CAD build for the part. Positions are in the model's coordinates, mm. Face numbers are marked on the shaded views. Round coordinates to 2 decimals unless told otherwise and drop trailing zeros. Loops run counter-clockwise (first coordinate to the right, second up) from the corner with the lowest first, then second, coordinate; pieces in that order, holes last. Notation, with made-up numbers: M 69.25,27 L 87.25,27 A16 ccw 87.25,32 Z; hole C 49.5,-28 d8. An arc over 180 degrees is marked long. Use a Markdown table: item, result. Add a question column.
(1) Band-saw the part on B-B, the plane y = 19. Write the cut outline in (x, z) (3 decimals), and give its area (3 significant figures).
(2) Wall check: L1, parallel to Y at x = -1, z = -1.5 (3 decimals); L2, parallel to Y at x = 0, z = -3.5; L3, parallel to X at y = 46.5, z = -0.75. Give the ranges that are in metal, low to high.
(3) Flat gauge pins, fed straight in: P1, Ø2, axis at y = 31.5, z = 1.5, coming from the -X side; P2, Ø1, axis at y = 34, z = 2, coming from the +X side; P3, Ø5, axis at x = -3, y = 29.5, coming from the -Z side. Where does each tip first touch, or does it go through?
(4) Two-plate mould, pull along X, no slides. Class the marked faces 1, 2, 3 and 4: released by +X, released by -X, zero draft, split by the parting line, or undercut.
Autodesk Inventor part; units mm, degrees
ref_plane "YZ Plane" through (0, 0, 0) normal (1, 0, 0) x (0, 1, 0)
ref_plane "XZ Plane" through (0, 0, 0) normal (0, 1, 0) x (-1, 0, 0)
ref_plane "XY Plane" through (0, 0, 0) normal (0, 0, 1) x (1, 0, 0)
sketch "Sketch1" plane through (0, 0, 0) normal (0, 1, 0) x (-1, 0, 0)
  circle A0 centre (0, 0) radius 3.175
  dimension "d0" = 6.35
extrude "Extrusion1" add sketch "Sketch1" along normal blind 50.8
sketch "Sketch2" plane through (0, 50.8, 0) normal (0, 1, 0) x (1, 0, 0)
  circle A0 centre (0, 0) radius 3.175
  circle A1 centre (0, 0) radius 4.7625
  dimension "d3" = 9.525
extrude "Extrusion2" add sketch "Sketch2" along normal blind 6.35 contours A0 | A1
sketch "Sketch3" plane through (0, 57.15, 0) normal (0, 1, 0) x (1, 0, 0)
  circle A0 centre (0, 0) radius 4.7625
  line L0 (-1.3748, 2.3812) -> (1.3748, 2.3813)
  line L1 (1.3748, 2.3813) -> (2.7496, 0)
  line L2 (2.7496, 0) -> (1.3748, -2.3813)
  line L3 (1.3748, -2.3813) -> (-1.3748, -2.3813)
  line L4 (-1.3748, -2.3813) -> (-2.7496, 0)
  line L5 (-2.7496, 0) -> (-1.3748, 2.3812)
  dimension "d6" = 4.7625
extrude "Extrusion3" cut sketch "Sketch3" against normal blind 3.175 contours L0 L1 L2 L3 L4 L5
fillet "Fillet1" radius 0.3969 3 edges at (3.175, 50.8, 0) (-4.7625, 57.15, 0) (3.175, 0, 0)
properties part number "Bolt_0.25_20_2.0len_SocketHead" material "Stainless Steel, Austenitic"
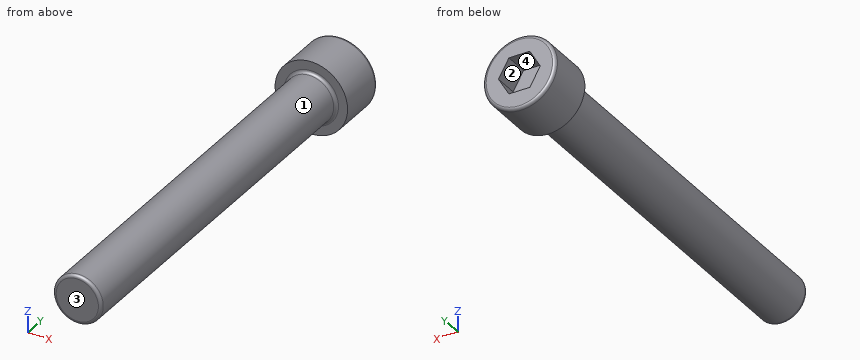
Return value:
| question | item | result |
|---|---|---|
| 1 | outline | C 0,0 d6.35 |
| 1 | area | 31.7 mm^2 |
| 2 | L1 | 0 to 53.975 |
| 2 | L2 | 50.79 to 57.15 |
| 2 | L3 | -3.09 to 3.09 |
| 3 | P1 | x = -3.14 |
| 3 | P2 | x = 2.8 |
| 3 | P3 | z = -3.14 |
| 4 | face 1 | split by the parting line |
| 4 | face 2 | undercut |
| 4 | face 3 | zero draft |
| 4 | face 4 | undercut |
